Geometry: final body of the model. Coordinates: model frame, mm. Give positions to 0.01 mm unless a question says otherwise; leave off trailing zeros. Write each loop counter-clockwise with the first axis right and the second up, starting at its lowest first coordinate (ties: lowest second). Pieces come first, ordered by that corner, then holes. Notation, with made-up numbers: M 11.25,82.5 L 42.25,82.5 A26 ccw 42.25,99.5 Z; hole C 68.25,75.5 d1. An arc over 180 degrees is marked long. Use one line per item in the form item = value. Start each with the question number.
Item 1: Contact query for a flat-ended pin moving along its axis: P1, Ø6, axis at x = 10.5, z = 151.5, coming from the -Y side. Output: stop coordinate, or through.
Item 2: Section query B-B on x = 13.5. Return loops of the section in (y, z).
Item 3: Section query C-C on z = 368.5. Return loops of the section in (x, y), then the cut area to 3 significant figures.
Item 4: Section query A-A on y = -255.5. Return loops of the section in (x, z).
Item 5: Material intervals for line 1 along Z through (x, y) = (4, -878); line 2 along Y through (x, z) = (8.5, 46.5), sorted ascending. Write a range as from..to.
from build123d import *

# Parameters (mm, degrees)
BOSS_EXTRUDE1_DEPTH = 20


with BuildPart() as part:
    # Sketch1 → Boss-Extrude1 (new body)
    with BuildSketch(Plane(origin=(0, 0, 0), x_dir=(0, 0, -1), z_dir=(1, 0, 0))):
        Polygon((-600, -650), (-600, -520), (0, -520), (0, -650), (0, -670), (0, -1300), (20, -1300), (20, -500), (20, 0), (20, 250), (0, 250), (-600, 250), (-620, 250), (-620, 0), (-620, -500), (-620, -1300), (-600, -1300), (-600, -670), align=None)
        Polygon((0, 230), (0, 0), (0, -500), (-600, -500), (-600, 0), (-600, 230), align=None, mode=Mode.SUBTRACT)
    extrude(amount=BOSS_EXTRUDE1_DEPTH)


solid = part.part
Answer sheet:
q1.P1 = -520
q2.outline = M -1300,-20 L 250,-20 L 250,620 L -1300,620 L -1300,600 L -520,600 L -520,0 L -1300,0 Z; hole M -500,0 L 230,0 L 230,600 L -500,600 Z
q3.outline = M 0,-520 L 20,-520 L 20,-500 L 0,-500 Z; M 0,230 L 20,230 L 20,250 L 0,250 Z
q3.area = 800 mm2
q4.outline = M 0,-20 L 20,-20 L 20,0 L 0,0 Z; M 0,600 L 20,600 L 20,620 L 0,620 Z
q5.line_1 = -20..0, 600..620
q5.line_2 = -520..-500, 230..250
